```python
from build123d import *

# Parameters (mm, degrees)
SKETCH1_R           = 1.5
BOSS_EXTRUDE1_DEPTH = 1.75
CHAMFER1_SIZE       = 1.5


with BuildPart() as part:
    # Sketch1 → Boss-Extrude1 (new body)
    with BuildSketch(Plane(origin=(0, 0, 0), x_dir=(1, 0, 0), z_dir=(0, 1, 0))):
        with BuildLine():
            Line((8, 0), (8, 47))
            Line((8, 47), (9.5, 50))
            Line((9.5, 50), (9.5, 58.7))
            ThreePointArc((9.5, 58.7), (8.328427125, 61.528427125), (5.5, 62.7))
            Line((5.5, 62.7), (-5.5, 62.7))
            ThreePointArc((-5.5, 62.7), (-8.328427125, 61.528427125), (-9.5, 58.7))
            Line((-9.5, 58.7), (-9.5, 50))
            Line((-9.5, 50), (-8, 47))
            Line((-8, 47), (-8, 0))
            Line((-8, 0), (-8, -2.5))
            ThreePointArc((-8, -2.5), (-9.171572875, -5.328427125), (-12, -6.5))
            Line((-12, -6.5), (-39, -6.5))
            ThreePointArc((-39, -6.5), (-41.828427125, -7.671572875), (-43, -10.5))
            Line((-43, -10.5), (-43, -56))
            Line((-43, -56), (-43, -56.3))
            ThreePointArc((-43, -56.3), (-41.242640687, -60.542640687), (-37, -62.3))
            Line((-37, -62.3), (-35, -62.3))
            ThreePointArc((-35, -62.3), (-32.171572875, -61.128427125), (-31, -58.3))
            Line((-31, -58.3), (-31, -58))
            ThreePointArc((-31, -58), (-30.414213562, -56.585786438), (-29, -56))
            Line((-29, -56), (19.5, -56))
            ThreePointArc((19.5, -56), (21.621320344, -56.878679656), (22.5, -59))
            Line((22.5, -59), (22.5, -59.3))
            ThreePointArc((22.5, -59.3), (23.378679656, -61.421320344), (25.5, -62.3))
            Line((25.5, -62.3), (26, -62.3))
            ThreePointArc((26, -62.3), (28.121320344, -61.421320344), (29, -59.3))
            Line((29, -59.3), (29, -56))
            Line((29, -56), (29, -8.5))
            ThreePointArc((29, -8.5), (28.414213562, -7.085786438), (27, -6.5))
            Line((27, -6.5), (12, -6.5))
            ThreePointArc((12, -6.5), (9.171572875, -5.328427125), (8, -2.5))
            Line((8, -2.5), (8, 0))
        make_face()
        with Locations(Location((0, 0, 0), (0, 0, 270))):
            Circle(SKETCH1_R, mode=Mode.SUBTRACT)
        with Locations(Location((0, 55.5, 0), (0, 0, 270))):
            Circle(SKETCH1_R, mode=Mode.SUBTRACT)
        with Locations(Location((25, -16.5, 0), (0, 0, 270))):
            Circle(SKETCH1_R, mode=Mode.SUBTRACT)
        with Locations(Location((25, -51.5, 0), (0, 0, 270))):
            Circle(SKETCH1_R, mode=Mode.SUBTRACT)
        with Locations(Location((-36.5, -16.5, 0), (0, 0, 270))):
            Circle(SKETCH1_R, mode=Mode.SUBTRACT)
        with Locations(Location((-36.5, -49.5, 0), (0, 0, 270))):
            Circle(SKETCH1_R, mode=Mode.SUBTRACT)
        with BuildLine():
            Line((-31, -22.5), (-31, -44))
            ThreePointArc((-31, -44), (-30.414213562, -45.414213562), (-29, -46))
            Line((-29, -46), (20.5, -46))
            ThreePointArc((20.5, -46), (21.914213562, -45.414213562), (22.5, -44))
            Line((22.5, -44), (22.5, -22.5))
            ThreePointArc((22.5, -22.5), (21.914213562, -21.085786438), (20.5, -20.5))
            Line((20.5, -20.5), (-29, -20.5))
            ThreePointArc((-29, -20.5), (-30.414213562, -21.085786438), (-31, -22.5))
        make_face(mode=Mode.SUBTRACT)
    extrude(amount=BOSS_EXTRUDE1_DEPTH)

    # Chamfer1
    chamfer1_edges = [part.edges().sort_by_distance(p)[0] for p in [
        (25, 0, 15),
        (25, 0, 50),
        (-36.5, 0, 15),
        (-36.5, 0, 48),
        (0, 0, -1.5),
        (0, 0, -57),
    ]]
    chamfer(chamfer1_edges, length=CHAMFER1_SIZE)


solid = part.part
```
For this review, take the finished solid that the model builds, in its own axes (mm). A direction names the side the tool comes from. Round coordinates to 2 decimals unless told otherwise and drop trailing zeros. Loops run counter-clockwise (first coordinate to the right, second up) from the corner with the lowest first, then second, coordinate; pieces in that order, holes last.
(1) Mouldability with a two-part tool opening along X and no side actions: class faces 4 (the cylindrical face through (-32.203, 0.863, 61.159)), 5 (the flat face through (-8, 1.75, 13)), 6 (the cylindrical face through (-41.289, 0.863, 60.496)) as released by +X, released by -X, zero draft, split by the parting line, or undercut.
Returned:
face 4: undercut
face 5: zero draft
face 6: released by -X
(2) We need section A-A (z = 34). Give the boundary of the cut face in (x, y), plus the area to 3 significant figures.
Returned:
outline: (-43, 0) - (-31, 0) - (-31, 1.75) - (-43, 1.75) - close; (22.5, 0) - (29, 0) - (29, 1.75) - (22.5, 1.75) - close
area: 32.4 mm2
(3) Tool access review of faces 1 (the cylindrical face through (-9.141, 0.863, 5.297)), 2 (the conical face through (-2, 1, 0)), 3 (the cylindrical face through (21.6, 0.86, 56.86)): name each direction out of +Z, -Z, +X, -X, +Y, -Y from which nothing blocks a thin tool from reaching the whole face with its end or side.
Returned:
face 1: -X, +Y, -Y
face 2: -Y
face 3: +Z, +Y, -Y
(4) Wall thickness on line 1 along X through (y, z) = (1.6, 16.5); line 2 along Z through (x, y) = (12, 0.9); line 3 along X through (y, z) = (1.6, -55.5): over which ranges is each line inside the solid? List them lowest first.
Returned:
line 1: x = -43 to -38, -35 to 23.5, 26.5 to 29
line 2: z = 6.5 to 20.5, 46 to 56
line 3: x = -9.5 to -1.5, 1.5 to 9.5
(5) Clearance check with flat-ended pins moving along their axes: P1, Ø0.5, axis at y = 1, z = -53, coming from the +X side; P2, Ø0.9, axis at x = -19.5, y = 0.5, coming from the -Z side; P3, Ø0.5, axis at y = 0.5, z = -27, coming from the -X side. State where each tip first meets the part, or that it passes through.
Returned:
P1: stops at x = 9.5
P2: stops at z = 6.5
P3: stops at x = -8
(6) We need section C-C (x = -16.5). Give the boundary of the cut face in (y, z), plus the area to 3 significant figures.
Returned:
outline: (0, 6.5) - (1.75, 6.5) - (1.75, 20.5) - (0, 20.5) - close; (0, 46) - (1.75, 46) - (1.75, 56) - (0, 56) - close
area: 42.0 mm2
(7) We need section D-D (z = 0). Give the boundary of the cut face in (x, y), plus the area to 3 significant figures.
Returned:
outline: (-8, 0) - (-3, 0) - (-1.5, 1.5) - (-1.5, 1.75) - (-8, 1.75) - close; (1.5, 1.5) - (3, 0) - (8, 0) - (8, 1.75) - (1.5, 1.75) - close
area: 20.5 mm2
(8) We need section B-B (x = 0). Give the boundary of the cut face in (y, z), plus the area to 3 significant figures.
Returned:
outline: (0, -62.7) - (1.75, -62.7) - (1.75, -57) - (1.5, -57) - (0, -58.5) - close; (0, -52.5) - (1.5, -54) - (1.75, -54) - (1.75, -1.5) - (1.5, -1.5) - (0, -3) - close; (0, 3) - (1.5, 1.5) - (1.75, 1.5) - (1.75, 20.5) - (0, 20.5) - close; (0, 46) - (1.75, 46) - (1.75, 56) - (0, 56) - close
area: 148 mm2
